```python
from build123d import *

# Parameters (mm, degrees)
F0_W     = 50
F0_H     = 50
F0_W_2   = 40
F0_H_2   = 40
F1_DEPTH = 50
F2_R     = 5
F3_R     = 3


with BuildPart() as f1:
    # F0 (on Front) → F1 (new body)
    with BuildSketch(Plane.XZ):
        Rectangle(F0_W, F0_H)
        Rectangle(F0_W_2, F0_H_2, mode=Mode.SUBTRACT)
    extrude(amount=F1_DEPTH)

    # F2
    f2_edges = [f1.edges().sort_by_distance(p)[0] for p in [
        (25, -25, 25),
        (-25, -25, 25),
        (25, -25, -25),
        (-25, -25, -25),
    ]]
    fillet(f2_edges, radius=F2_R)

    # F3
    f3_edges = [f1.edges().sort_by_distance(p)[0] for p in [
        (20, -25, 20),
        (-20, -25, 20),
        (-20, -25, -20),
        (20, -25, -20),
    ]]
    fillet(f3_edges, radius=F3_R)


solid = f1.part
```
CAD build for the part. Positions are in the model's coordinates, mm. A direction names the side the tool comes from. Coordinates: 2 decimals unless noted, no trailing zeros. Order: outer loops, then holes, each group sorted by start corner. A loop starts at its lowest first (then second) coordinate and runs counter-clockwise, first axis right, second up. Notation, with made-up numbers: (82, -34) - (109, -34) arc R36 ccw to (109, 0) - close; hole circle Ø3 at (-1.5, 71). An arc over 180 degrees is marked (long way). Use a Markdown table: item, result. Add a question column.
(1) Pull direction X, two halves, no side cores. Call faces 3 (the face through (25, -25, 0)), 4 (the face through (-19.1, -25.35, -19.14)), 5 (the face through (-23, 0, 0)): +X half, -X half, draft (parallel to the pull), parting line (faces both ways), or undercut.
(2) Saw through at A-A (z = -16). Give the cut face in (x, y).
(3) Saw through at C-C (y = -44.5). Give the cut face in (x, z).
(4) Drill centre lines: line 1 along X through (y, z) = (-7, -17); line 2 along Z through (x, y) = (-21, -13.5). Where is each one in solid material? Low to high. Write a range as [from, to].
(5) Saw through at B-B (x = 1). Give the cut face in (y, z), then the cut area to 3 significant figures.
(6) Which spindle directions (+Z, -Z, +X, -X, +Y, -Y) get a long thin tool onto all of the face, cutting with end or side? Do faces 1 (the face through (0, -25, 20)), 2 (the face through (23, -25, -24)). Say none if no direction does.
Solved:
| question | item | result |
|---|---|---|
| 1 | face 3 | +X half |
| 1 | face 4 | undercut |
| 1 | face 5 | draft |
| 2 | outline | (-25, -50) - (-20, -50) - (-20, 0) - (-25, 0) - close; (20, -50) - (25, -50) - (25, 0) - (20, 0) - close |
| 3 | outline | (-25, -20) arc R5 ccw to (-20, -25) - (20, -25) arc R5 ccw to (25, -20) - (25, 20) arc R5 ccw to (20, 25) - (-20, 25) arc R5 ccw to (-25, 20) - close; hole (-20, -17) arc R3 ccw to (-17, -20) - (17, -20) arc R3 ccw to (20, -17) - (20, 17) arc R3 ccw to (17, 20) - (-17, 20) arc R3 ccw to (-20, 17) - close |
| 4 | line 1 | x = [-25, -20], [20, 25] |
| 4 | line 2 | z = [-24.9, 24.9] |
| 5 | outline | (-50, -25) - (0, -25) - (0, -20) - (-50, -20) - close; (-50, 20) - (0, 20) - (0, 25) - (-50, 25) - close |
| 5 | area | 500 mm² |
| 6 | face 1 | +Y, -Y |
| 6 | face 2 | -Z, +X, +Y, -Y |
